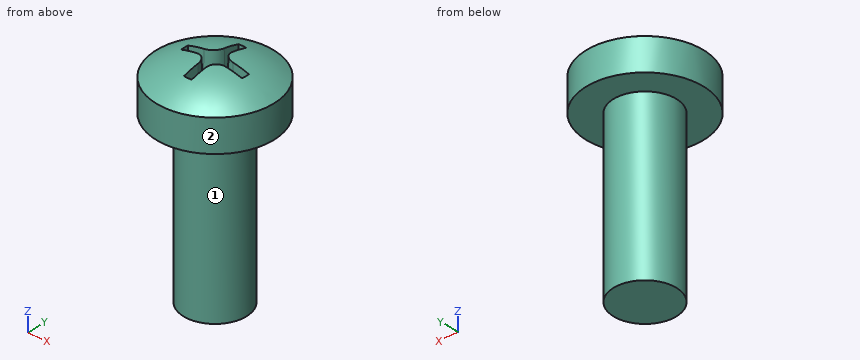
```python
from build123d import *

# Parameters (mm, degrees)
SKETCH1_R          = 1.5
BASE_EXTRUDE_DEPTH = 8
CUT_EXTRUDE1_DEPTH = 1.799999969
CUT_EXTRUDE1_TAPER = 2


with BuildPart() as part:
    # Sketch1 → Base-Extrude (new body)
    with BuildSketch(Plane.XY):
        Circle(SKETCH1_R)
    extrude(amount=BASE_EXTRUDE_DEPTH)

    # Sketch6 → Boss-Revolve2 (revolve)
    with BuildSketch(Plane(origin=(0, 0, 0), x_dir=(1, 0, 0), z_dir=(0, 1, 0))):
        with BuildLine():
            Line((0, -8), (2.7999999, -8))
            Line((2.7999999, -8), (2.7999999, -9.54246308))
            ThreePointArc((2.7999999, -9.54246308), (1.46418655, -10.180811406), (0, -10.4))
            Line((0, -10.4), (0, -8))
        make_face()
    revolve(axis=Axis((0, 0, -0.393620135), (0, 0, 1)))

    # Sketch7 → Cut-Extrude1 (cut)
    with BuildSketch(Plane(origin=(0, 0, 10.7000001), x_dir=(-1, 0, 0), z_dir=(0, 0, -1))):
        with BuildLine():
            ThreePointArc((0.205000004, 1.48592565), (0, 1.500000013), (-0.205000004, 1.48592565))
            Line((-0.205000004, 1.48592565), (-0.205000004, 0.708178558))
            ThreePointArc((-0.205000004, 0.708178558), (-0.35072876, 0.355344481), (-0.702967546, 0.208182689))
            Line((-0.702967546, 0.208182689), (-1.48592565, 0.205000004))
            ThreePointArc((-1.48592565, 0.205000004), (-1.500000013, 0), (-1.48592565, -0.205000004))
            Line((-1.48592565, -0.205000004), (-0.702967546, -0.208182689))
            ThreePointArc((-0.702967546, -0.208182689), (-0.35072876, -0.355344481), (-0.205000004, -0.708178558))
            Line((-0.205000004, -0.708178558), (-0.205000004, -1.48592565))
            ThreePointArc((-0.205000004, -1.48592565), (0, -1.500000013), (0.205000004, -1.48592565))
            Line((0.205000004, -1.48592565), (0.205000004, -0.708178558))
            ThreePointArc((0.205000004, -0.708178558), (0.35072876, -0.355344481), (0.702967546, -0.208182689))
            Line((0.702967546, -0.208182689), (1.48592565, -0.205000004))
            ThreePointArc((1.48592565, -0.205000004), (1.500000013, 0), (1.48592565, 0.205000004))
            Line((1.48592565, 0.205000004), (0.702967546, 0.208182689))
            ThreePointArc((0.702967546, 0.208182689), (0.35072876, 0.355344481), (0.205000004, 0.708178558))
            Line((0.205000004, 0.708178558), (0.205000004, 1.48592565))
        make_face()
    extrude(amount=CUT_EXTRUDE1_DEPTH, taper=CUT_EXTRUDE1_TAPER, mode=Mode.SUBTRACT)


solid = part.part
```
For this review, take the finished solid that the model builds, in its own axes (mm). Face numbers are marked on the shaded views. A direction names the side the tool comes from. Give positions to 0.01 mm unless a question says otherwise; leave off trailing zeros. Order: outer loops, then holes, each group sorted by start corner. A loop starts at its lowest first (then second) coordinate and runs counter-clockwise, first axis right, second up.
1) Take a section at B-B (y = -1.7). Give the boundary of the cut face in (x, z).
2) Insertion check: pin 1 (1.5 mm diameter, centred on y = 1.5, z = 5, fed in from -X). The pin has a flat end and moves straight along its axis. Give the tip position at first contact, or say it passes through.
3) Take a section at A-A (z = 5). Give the boundary of the cut face in (x, y), then the cut area to 3 significant figures.
4) Wall thickness on line 1 (X direction, y = 0.35, z = 9.25); line 2 (Y direction, x = 0.3, z = 2.25); line 3 (X direction, y = 0.1, z = 4): over which ranges is each line inside the solid? List them lowest first.
5) For the marked faces 1 and 2, list the 3-axis set-ups (+Z, -Z, +X, -X, +Y, -Y) from which the entire face can be reached by the end or side of a thin tool; tool diameter is ignored.
Derived:
1. outline: (-2.22, 8) - (2.22, 8) - (2.22, 9.54) arc R4.7 ccw to (-2.22, 9.54) - close
2. pin 1: stops at x = -1.3
3. outline: circle Ø3 at (0, 0)
3. area: 7.07 mm2
4. line 1: x = -2.78 to -0.29, 0.29 to 2.78
4. line 2: y = -1.47 to 1.47
4. line 3: x = -1.5 to 1.5
5. face 1: -Z
5. face 2: +Z, -Z
